Here's how the part is built. I have some questions about the finished solid (model axes, mm). A direction names the side the tool comes from. Coordinates: 2 decimals unless noted, no trailing zeros. Write each loop counter-clockwise with the first axis right and the second up, starting at its lowest first coordinate (ties: lowest second). Pieces come first, ordered by that corner, then holes.
```python
from build123d import *

# Parameters (mm, degrees)
F0_R     = 5
F1_DEPTH = 258
F2_R     = 9
F2_R_2   = 4
F3_DEPTH = 8
F4_R     = 5
F4_R_2   = 4
F5_DEPTH = 8


with BuildPart() as f1:
    # F0 (on Front) → F1 (new body, symmetric)
    with BuildSketch(Plane.XZ):
        Circle(F0_R)
    extrude(amount=F1_DEPTH, both=True)

    # F2 (on face) → F3 (cut)
    with BuildSketch(Plane.XZ.offset(258)):
        Circle(F2_R)
        Circle(F2_R_2, mode=Mode.SUBTRACT)
    extrude(amount=-F3_DEPTH, mode=Mode.SUBTRACT)

    # F4 (on face) → F5 (cut)
    with BuildSketch(Plane(origin=(0, 258, 0), x_dir=(-1, 0, 0), z_dir=(0, 1, 0))):
        Circle(F4_R)
        Circle(F4_R_2, mode=Mode.SUBTRACT)
    extrude(amount=-F5_DEPTH, mode=Mode.SUBTRACT)


solid = f1.part
```
1) Imagine slicing it at A-A on z = 2.25. Please give me the cut outline in (x, y), then the cut area to 3 significant figures.
Values follow:
outline: (-4.47, -250) - (-3.31, -250) - (-3.31, -258) - (3.31, -258) - (3.31, -250) - (4.47, -250) - (4.47, 250) - (3.31, 250) - (3.31, 258) - (-3.31, 258) - (-3.31, 250) - (-4.47, 250) - close
area: 4,570 mm2
2) On a 3-axis mill with a long thin cutter (end or side, diameter ignored), from which of +Z, -Z, +X, -X, +Y, -Y can I reach the whole of each face in a straight line? I mean faces 1 (the face through (0.867, 254.056, -3.905)), 2 (the face through (-1.08, -3.5, -4.88)), 3 (the face through (-0.867, -254.056, -3.905)). Say none if no direction works.
Values follow:
face 1: +Y
face 2: +Y, -Y
face 3: -Y
3) Will these pins go through, and if not, where does the flat tip stop? pin 1 (3 mm diameter, centred on x = -3.5, y = 128, fed in from -Z); pin 2 (5 mm diameter, centred on x = -3, y = 131.5, fed in from -Z).
Values follow:
pin 1: stops at z = -4.58
pin 2: stops at z = -4.97
4) I need wall thicknesses on probe 1 along X at (y, z) = (-232, -0.75); probe 2 along Y at (x, z) = (-3.5, -3.5); probe 3 along Z at (x, y) = (0.5, -116). Which ranges of each line are inside material? Lowest first, please.
Values follow:
probe 1: x = -4.94 to 4.94
probe 2: y = -250 to 250
probe 3: z = -4.97 to 4.97
5) Imagine slicing it at B-B on x = 0.75. Please give me the cut outline in (y, z).
Values follow:
outline: (-258, -3.93) - (-250, -3.93) - (-250, -4.94) - (250, -4.94) - (250, -3.93) - (258, -3.93) - (258, 3.93) - (250, 3.93) - (250, 4.94) - (-250, 4.94) - (-250, 3.93) - (-258, 3.93) - close
6) Imagine slicing it at C-C on y = -213. Please give me the cut outline in (x, z).
Values follow:
outline: circle Ø10 at (0, 0)
